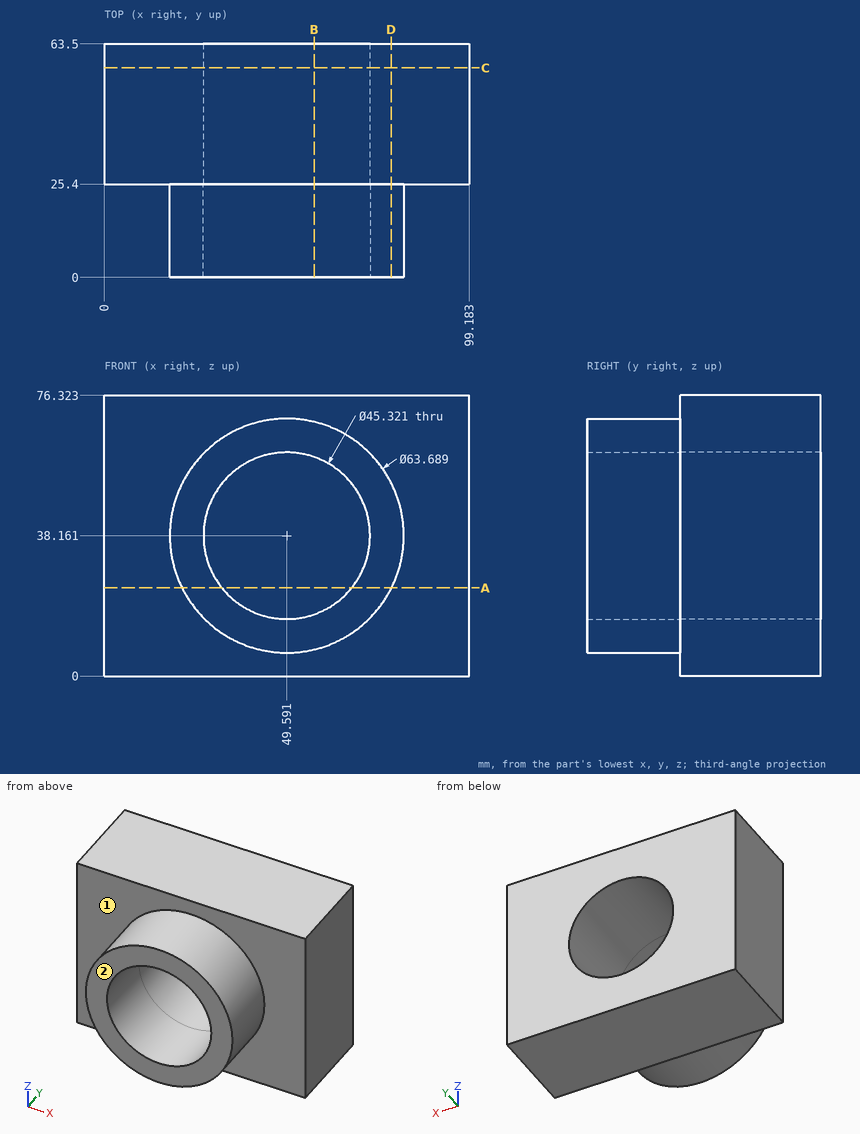
Could you check a few things on this drawing? It's one solid part, dimensions in mm from its lowest x, y, z. A direction names the side the tool comes from. Give positions to 0.01 mm unless a question says otherwise; leave off trailing zeros. Loops run counter-clockwise (first coordinate to the right, second up) from the corner with the lowest first, then second, coordinate; pieces in that order, holes last. Notation, with made-up numbers: (-29, 43) -> (-21, 43) arc R17 ccw to (-21, 72) -> close; hole circle Ø6 at (21.25, -36). An arc over 180 degrees is marked (long way). Use one line per item in the form item = value. Start each with the question number.
1) For P1, Ø2, axis at y = 17.5, z = 22.5, coming from the -X side, with a flat end and sliding along its axis, tell me the tip position at first contact or that it passes through.
2) Please list where these lines run through material, in increasing order: line 1 along Y through (x, z) = (5, 41.5); line 2 along X through (y, z) = (13, 58) (1 decimal); line 3 along Z through (x, y) = (50.5, 32).
3) Imagine slicing it at A-A (z = 24). Please give me the cut outline in (x, y), then the cut area to 3 significant figures.
4) Imagine slicing it at B-B (x = 57). Please give me the cut outline in (y, z).
5) Imagine slicing it at D-D (x = 78). Please give me the cut outline in (y, z).
6) Imagine slicing it at C-C (y = 57). Please give me the cut outline in (x, z).
7) Which directions (+Z, -Z, +X, -X, +Y, -Y) give clear straight access to the entire face, cutting with the end or side of a thin tool? Please do the marked faces 1 and 2.
Check values:
q1.P1 = 21.32
q2.line_1 = 25.4 to 63.5
q2.line_2 = 24.7 to 38.6, 60.5 to 74.5
q2.line_3 = 0 to 15.52, 60.8 to 76.32
q3.outline = (0, 25.4) -> (21.07, 25.4) -> (21.07, 0) -> (31.9, 0) -> (31.9, 63.5) -> (0, 63.5) -> close; (67.28, 0) -> (78.11, 0) -> (78.11, 25.4) -> (99.18, 25.4) -> (99.18, 63.5) -> (67.28, 63.5) -> close
q3.area = 2,980 mm^2
q4.outline = (0, 7.19) -> (25.4, 7.19) -> (25.4, 0) -> (63.5, 0) -> (63.5, 16.75) -> (0, 16.75) -> close; (0, 59.58) -> (63.5, 59.58) -> (63.5, 76.32) -> (25.4, 76.32) -> (25.4, 69.13) -> (0, 69.13) -> close
q5.outline = (0, 23.77) -> (25.4, 23.77) -> (25.4, 0) -> (63.5, 0) -> (63.5, 76.32) -> (25.4, 76.32) -> (25.4, 52.55) -> (0, 52.55) -> close
q6.outline = (0, 0) -> (99.18, 0) -> (99.18, 76.32) -> (0, 76.32) -> close; hole circle Ø45.32 at (49.59, 38.16)
q7.face_1 = -Y
q7.face_2 = +Z, -Z, +X, -X, -Y
